Design review of the part built by this model. Coordinates are the model's own, in mm. Face numbers are marked on the shaded views. A direction names the side the tool comes from. Coordinates: 2 decimals unless noted, no trailing zeros. Write each loop counter-clockwise with the first axis right and the second up, starting at its lowest first coordinate (ties: lowest second). Pieces come first, ordered by that corner, then holes. Notation, with made-up numbers: (49, 44) - (95, 44) arc R23 ccw to (95, 55) - close; hole circle Ø5 at (74, 1.25). An arc over 180 degrees is marked (long way). Use a Markdown table: item, result.
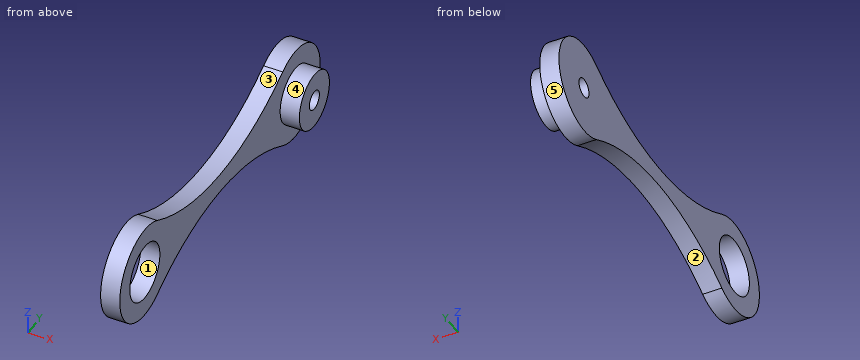
from build123d import *

# Parameters (mm, degrees)
SKETCH1_R           = 15
BOSS_EXTRUDE1_DEPTH = 10
SKETCH2_R           = 15
BOSS_EXTRUDE2_DEPTH = 10
SKETCH3_R           = 5
CUT_EXTRUDE1_DEPTH  = 45


with BuildPart() as part:
    # Sketch1 → Boss-Extrude1 (new body)
    with BuildSketch(Plane(origin=(0, 0, 0), x_dir=(0, 0, -1), z_dir=(1, 0, 0))):
        with BuildLine():
            ThreePointArc((21.680497925, -12.44813278), (0, 25), (-21.680497925, -12.44813278))
            ThreePointArc((-21.680497925, -12.44813278), (-5, -75), (-21.680497925, -137.55186722))
            ThreePointArc((-21.680497925, -137.55186722), (0, -175), (21.680497925, -137.55186722))
            ThreePointArc((21.680497925, -137.55186722), (5, -75), (21.680497925, -12.44813278))
        make_face()
        with Locations((0, -150)):
            Circle(SKETCH1_R, mode=Mode.SUBTRACT)
    extrude(amount=BOSS_EXTRUDE1_DEPTH)

    # Sketch2 → Boss-Extrude2 (add)
    with BuildSketch(Plane(origin=(10, 0, 0), x_dir=(0, 0, -1), z_dir=(1, 0, 0))):
        Circle(SKETCH2_R)
    extrude(amount=BOSS_EXTRUDE2_DEPTH)

    # Sketch3 → Cut-Extrude1 (cut)
    with BuildSketch(Plane(origin=(20, 0, 0), x_dir=(0, 0, -1), z_dir=(1, 0, 0))):
        Circle(SKETCH3_R)
    extrude(amount=-CUT_EXTRUDE1_DEPTH, mode=Mode.SUBTRACT)


solid = part.part
(1) For pin 1 (6 mm diameter, centred on x = 5, z = 7, fed in from +Y); pin 2 (2 mm diameter, centred on x = 3, y = -75.5, fed in from +Z); pin 3 (4 mm diameter, centred on x = 6, y = -154.5, fed in from +Z), all flat-tipped, find the tip position at first contact; note any pin that passes through.
Determined:
| item | result |
|---|---|
| pin 1 | y = 24.68 |
| pin 2 | z = 5.01 |
| pin 3 | z = 24.87 |
(2) Take a section at B-B on z = 0. Write out the cut boundary in (x, y), and give its area (3 significant figures).
Determined:
| item | result |
|---|---|
| outline | (0, -175) - (10, -175) - (10, -165) - (0, -165) - close; (0, -135) - (10, -135) - (10, -15) - (20, -15) - (20, -5) - (0, -5) - close; (0, 5) - (20, 5) - (20, 15) - (10, 15) - (10, 25) - (0, 25) - close |
| area | 1,800 mm2 |
(3) Take a section at C-C on x = 2.25. State how many separate pieces and enclosed holes the cut face has, and give its area (3 significant figures).
Determined:
| item | result |
|---|---|
| separate pieces | 1 |
| enclosed holes | 2 |
| area | 4,970 mm2 |
(4) For L1, parallel to Y at x = 15.25, z = 0; L2, parallel to Z at x = 6.25, y = -151; L3, parallel to X at y = -114.5, z = 6.5, list the stretches that pass through material, from the lowest coordinate up. Write a range as from..to.
Determined:
| item | result |
|---|---|
| L1 | -15..-5, 5..15 |
| L2 | -24.98..-14.97, 14.97..24.98 |
| L3 | 0..10 |
(5) Take a section at A-A on y = 0. Write out the cut boundary in (x, z).
Determined:
| item | result |
|---|---|
| outline | (0, -25) - (10, -25) - (10, -15) - (20, -15) - (20, -5) - (0, -5) - close; (0, 5) - (20, 5) - (20, 15) - (10, 15) - (10, 25) - (0, 25) - close |
(6) Take a section at D-D on z = 19.5. Write out the cut boundary in (x, y), and give its area (3 significant figures).
Determined:
| item | result |
|---|---|
| outline | (0, -165.64) - (10, -165.64) - (10, -133.59) - (0, -133.59) - close; (0, -16.41) - (10, -16.41) - (10, 15.64) - (0, 15.64) - close |
| area | 641 mm2 |
(7) Draft analysis for pull direction Z (two halves, no side actions). For the marked faces 1, 2 and 3, state which applies: +Z half, -Z half, draft (parallel to the pull), parting line (faces both ways), or undercut.
Determined:
| item | result |
|---|---|
| face 1 | undercut |
| face 2 | -Z half |
| face 3 | +Z half |
(8) Machinability: for the marked faces 4 and 5, which of the approach directions +Z, -Z, +X, -X, +Y, -Y give a long, thin tool a straight path to every point of the face, cutting with its end or side? Answer none if there is none.
Determined:
| item | result |
|---|---|
| face 4 | +X |
| face 5 | +X, -X |
